```python
from build123d import *

# Parameters (mm, degrees)
EXTRUDE_1_DEPTH     = 80
SKETCH_2_R          = 1.6
CUT_EXTRUDE_1_DEPTH = 50
SKETCH_5_R          = 1.6
CUT_EXTRUDE_2_DEPTH = 50
SKETCH_9_W          = 10
SKETCH_9_H          = 62
SKETCH_9_W_2        = 20
CUT_EXTRUDE_6_DEPTH = 50
FILLET_1_R          = 1
FILLET_2_R          = 1
FILLET_3_R          = 1
FILLET_4_R          = 0.5
FILLET_5_R          = 0.5


with BuildPart() as part:
    # 草图1 → 凸台-拉伸1 (new body)
    with BuildSketch(Plane.XY):
        Polygon((5.79442956, 1.085282156), (17.784664248, -66.914717844), (26.784664248, -66.914717844), (26.784664248, -68.914717844), (16.106464985, -68.914717844), (4.116230297, -0.914717844), (-4.883769703, -0.914717844), (-4.883769703, 1.085282156), align=None)
    extrude(amount=EXTRUDE_1_DEPTH)

    # 草图2 → 切除-拉伸1 (cut)
    with BuildSketch(Plane(origin=(0, 1.085282156, 0), x_dir=(1, 0, 0), z_dir=(0, 1, 0))):
        with Locations(Location((-0.383769703, -20, 0), (0, 0, 270))):
            Circle(SKETCH_2_R)
        with Locations(Location((-0.383769703, -60, 0), (0, 0, 270))):
            Circle(SKETCH_2_R)
    extrude(amount=-CUT_EXTRUDE_1_DEPTH, mode=Mode.SUBTRACT)

    # 草图5 → 切除-拉伸2 (cut)
    with BuildSketch(Plane(origin=(0, -66.914717844, 0), x_dir=(1, 0, 0), z_dir=(0, 1, 0))):
        with Locations(Location((22.284664248, -10, 0), (0, 0, 270))):
            Circle(SKETCH_5_R)
        with Locations(Location((22.284664248, -70, 0), (0, 0, 270))):
            Circle(SKETCH_5_R)
    extrude(amount=-CUT_EXTRUDE_2_DEPTH, mode=Mode.SUBTRACT)

    # 草图9 → 切除-拉伸6 (cut)
    with BuildSketch(Plane(origin=(5.805300309, 1.023631076, 0), x_dir=(0, 0, -1), z_dir=(0.9848077530122086, 0.17364817766692736, 0))):
        with Locations((-75, -34.461902656)):
            Rectangle(SKETCH_9_W, SKETCH_9_H)
        with Locations((-55, -34.461902656)):
            Rectangle(SKETCH_9_W_2, SKETCH_9_H)
        with Locations((-25, -34.461902656)):
            Rectangle(SKETCH_9_W_2, SKETCH_9_H)
        with Locations((-5, -34.461902656)):
            Rectangle(SKETCH_9_W, SKETCH_9_H)
    extrude(amount=-CUT_EXTRUDE_6_DEPTH, mode=Mode.SUBTRACT)

    # 圆角1
    fillet_1_edges = [part.edges().sort_by_distance(p)[0] for p in [
        (16.106464985, -68.914717844, 40),
    ]]
    fillet(fillet_1_edges, radius=FILLET_1_R)

    # 圆角2
    fillet_2_edges = [part.edges().sort_by_distance(p)[0] for p in [
        (16.187832658, -63.617406365, 0),
        (5.421645643, -2.559325678, 0),
        (16.187832658, -63.617406365, 80),
        (5.421645643, -2.559325678, 80),
        (16.187832658, -63.617406365, 70),
        (16.187832658, -63.617406365, 65),
        (16.187832658, -63.617406365, 45),
        (16.187832658, -63.617406365, 35),
        (16.187832658, -63.617406365, 15),
        (16.187832658, -63.617406365, 10),
    ]]
    fillet(fillet_2_edges, radius=FILLET_2_R)

    # 圆角3
    fillet_3_edges = [part.edges().sort_by_distance(p)[0] for p in [
        (26.784664248, -67.914717844, 0),
        (26.784664248, -67.914717844, 80),
        (5.421645643, -2.559325678, 70),
        (5.421645643, -2.559325678, 65),
        (5.421645643, -2.559325678, 45),
        (5.421645643, -2.559325678, 35),
        (5.421645643, -2.559325678, 15),
        (5.421645643, -2.559325678, 10),
    ]]
    fillet(fillet_3_edges, radius=FILLET_3_R)

    # 圆角4
    fillet_4_edges = [part.edges().sort_by_distance(p)[0] for p in [
        (17.784664248, -66.914717844, 40),
    ]]
    fillet(fillet_4_edges, radius=FILLET_4_R)

    # 圆角5
    fillet_5_edges = [part.edges().sort_by_distance(p)[0] for p in [
        (4.116230297, -0.914717844, 40),
    ]]
    fillet(fillet_5_edges, radius=FILLET_5_R)


solid = part.part
```
Could you check a few things on this model? Use its own coordinates, in mm. A direction names the side the tool comes from. Coordinates: 2 decimals unless noted, no trailing zeros. Write each loop counter-clockwise with the first axis right and the second up, starting at its lowest first coordinate (ties: lowest second). Pieces come first, ordered by that corner, then holes. Notation, with made-up numbers: (-29.75, -31.5) -> (28.25, -31.5) arc R18 cw to (28.25, -10.5) -> close; hole circle Ø9 at (37.25, -28.75). An arc over 180 degrees is marked (long way). One line per question, with ' | ' between items. Start each with the question number.
1. Will these pins go through, and if not, where does the flat tip stop? P1, Ø3.5, axis at x = 11.5, y = -33, coming from the +Z side; P2, Ø8, axis at y = -17.5, z = 61.5, coming from the +X side; P3, Ø8, axis at x = 15, y = -49, coming from the -Z side; P4, Ø3.5, axis at x = 10, y = -46.5, coming from the -Z side (1 decimal).
2. Please list where these lines run through material, in increasing order: line 1 along X through (y, z) = (-68.2, 70); line 2 along Y through (x, z) = (-1.5, 37); line 3 along X through (y, z) = (-67.35, 10).
3. If we section it at B-B (y = -26.5): Please give me the cut outline in (x, z).
4. Thinking about a two-plate mould opening in X: for faces 1 (the face through (23.87, -67.9, 9.79)), 2 (the face through (-1, -0.915, 39)), 3 (the face through (5.435, -2.557, 55.126)), which applies, pulls with the +X half, pulls with the -X half, needs draft (parallel to the pull), parting line crosses it, or undercut?
5. If we section it at D-D (x = 13.5): Please give me the cut outline in (y, z), and give its area (3 significant figures).
6. If we section it at C-C (z = 60): Please give me the cut outline in (x, y), and give its area (3 significant figures).
7. For faces 4 (the face through (16.202, -63.615, 5.056)), 5 (the face through (16.202, -63.615, 25.126)), 6 (the face through (22, -66.915, 39)), 7 (the face through (5.435, -2.557, 5.056)), which set-ups out of +Z, -Z, +X, -X, +Y, -Y let a thin tool reach every point of the face, with its end or its side?
8. If we section it at A-A (z = 17.5): Please give me the cut outline in (x, y).
Return value:
1) P1: stops at z = 70 | P2: stops at x = 9.41 | P3: stops at z = 10 | P4: passes through
2) line 1: x = 15.99 to 20.68, 23.88 to 26.78 | line 2: y = -0.91 to 1.09 | line 3: x = 15.83 to 20.68, 23.88 to 26.78
3) outline: (8.63, 10) -> (10.66, 10) -> (10.66, 15) -> (8.63, 15) -> close; (8.63, 35) -> (10.66, 35) -> (10.66, 45) -> (8.63, 45) -> close; (8.63, 65) -> (10.66, 65) -> (10.66, 70) -> (8.63, 70) -> close
4) face 1: undercut | face 2: needs draft | face 3: pulls with the +X half
5) outline: (-54.13, 10) -> (-42.62, 10) -> (-42.62, 15) -> (-54.13, 15) -> close; (-54.13, 35) -> (-42.62, 35) -> (-42.62, 45) -> (-54.13, 45) -> close; (-54.13, 65) -> (-42.62, 65) -> (-42.62, 70) -> (-54.13, 70) -> close | area: 230 mm²
6) outline: (-4.88, -0.91) -> (-1.98, -0.91) -> (-1.98, 1.09) -> (-4.88, 1.09) -> close; (1.22, -0.91) -> (3.7, -0.91) arc R0.5 cw to (4.19, -1.33) -> (4.44, -2.73) -> (6.41, -2.39) -> (5.79, 1.09) -> (1.22, 1.09) -> close; (15.2, -63.79) -> (15.96, -68.09) arc R1 ccw to (16.95, -68.91) -> (26.78, -68.91) -> (26.78, -66.91) -> (18.2, -66.91) arc R0.5 cw to (17.71, -66.5) -> (17.17, -63.44) -> close | area: 47.0 mm²
7) face 4: -Z, -X, +Y | face 5: -X, +Y | face 6: +Z, -Z, +X, +Y | face 7: -Z, +X, -Y
8) outline: (-4.88, -0.91) -> (3.7, -0.91) arc R0.5 cw to (4.19, -1.33) -> (4.44, -2.73) -> (6.41, -2.39) -> (5.79, 1.09) -> (-4.88, 1.09) -> close; (15.2, -63.79) -> (15.96, -68.09) arc R1 ccw to (16.95, -68.91) -> (26.78, -68.91) -> (26.78, -66.91) -> (18.2, -66.91) arc R0.5 cw to (17.71, -66.5) -> (17.17, -63.44) -> close
